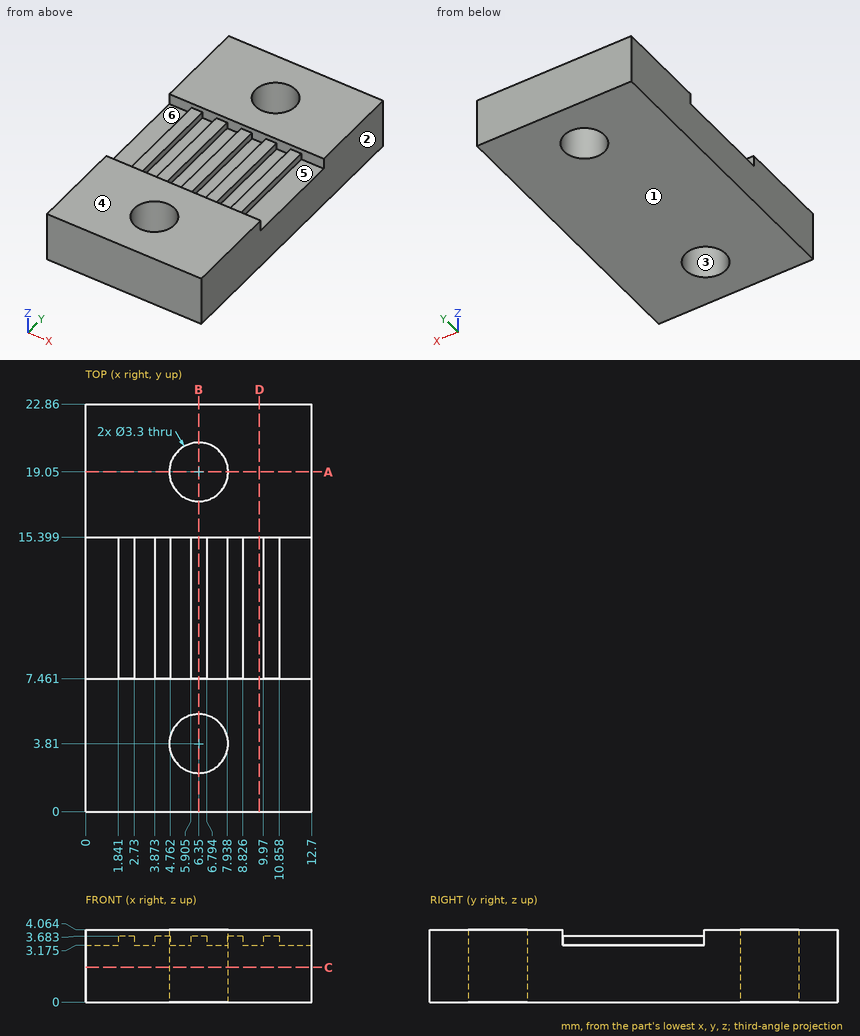
Can you work these out from the drawing? Everything is in mm from the part's minimum corner. A direction names the side the tool comes from. Coordinates: 2 decimals unless noted, no trailing zeros. Loops run counter-clockwise (first coordinate to the right, second up) from the corner with the lowest first, then second, coordinate; pieces in that order, holes last.
1. If we mould it in two halves opening along X, with no side actions, what happens to the marked faces 1, 2 and 3? For each: pulls with the +X half, pulls with the -X half, needs draft (parallel to the pull), parting line crosses it, or undercut.
2. For P1, Ø1.5, axis at x = 11.5, y = 12.5, coming from the +Z side; P2, Ø0.6, axis at x = 7.5, y = 13, coming from the +Z side (1 decimal), each with a flat end and sliding along its axis, tell me the tip position at first contact or that it passes through.
3. Imagine slicing it at D-D, the plane x = 9.75. Please give me the cut outline in (y, z) (1 decimal).
4. I need wall thicknesses on L1, parallel to Y at x = 6.35, z = 2.05; L2, parallel to X at y = 3.81, z = 2.7; L3, parallel to Y at x = 5.75, z = 2.2. Which ranges of each line are inside material? Lowest first, please.
5. Imagine slicing it at A-A, the plane y = 19.05. Please give me the cut outline in (x, z) (1 decimal).
6. Imagine slicing it at B-B, the plane x = 6.35. Count the separate pieces of the cut face and the enclosed holes in it.
7. For the marked faces 4, 5 and 6, which set-ups out of +Z, -Z, +X, -X, +Y, -Y let a thin tool reach every point of the face, with its end or its side?
8. Imagine slicing it at C-C, the plane z = 1.95. Please give me the cut outline in (x, y).
Taken from the geometry:
1. face 1: needs draft
1. face 2: pulls with the +X half
1. face 3: undercut
2. P1: stops at z = 3.68
2. P2: stops at z = 3.2
3. outline: (0, 0) - (22.9, 0) - (22.9, 4.1) - (15.4, 4.1) - (15.4, 3.2) - (7.5, 3.2) - (7.5, 4.1) - (0, 4.1) - close
4. L1: y = 0 to 2.16, 5.46 to 17.4, 20.7 to 22.86
4. L2: x = 0 to 4.7, 8 to 12.7
4. L3: y = 0 to 2.27, 5.35 to 17.51, 20.59 to 22.86
5. outline: (0, 0) - (4.7, 0) - (4.7, 4.1) - (0, 4.1) - close; (8, 0) - (12.7, 0) - (12.7, 4.1) - (8, 4.1) - close
6. separate pieces: 3
6. enclosed holes: 0
7. face 4: +Z, +X, -X, +Y, -Y
7. face 5: +Z, +X
7. face 6: +Z, -X
8. outline: (0, 0) - (12.7, 0) - (12.7, 22.86) - (0, 22.86) - close; hole circle Ø3.3 at (6.35, 3.81); hole circle Ø3.3 at (6.35, 19.05)
